Geometry check sheet. Reference: the model listing, model coordinates, mm. Face numbers are marked on the shaded views. A direction names the side the tool comes from. Coordinates: 2 decimals unless noted, no trailing zeros. Write each loop counter-clockwise with the first axis right and the second up, starting at its lowest first coordinate (ties: lowest second). Pieces come first, ordered by that corner, then holes. Notation, with made-up numbers: (-28, 35) -> (17, 35) arc R15 ccw to (17, 58) -> close; hole circle Ø10 at (-7.75, 45.25). An arc over 180 degrees is marked (long way). Answer in a Markdown table with one row per item. Add a question column.
1. Depth check by flat-ended pin: P1, Ø1.6, axis at y = 21, z = 21, coming from the +X side; P2, Ø0.6, axis at x = 15, z = 21.5, coming from the -Y side; P3, Ø0.9, axis at x = 35.5, y = 51.5, coming from the +Z side. Enter the tip coordinate at first touch or a pass-through.
2. Cross-section at A-A on z = 11. Record the cut outline in (x, y), and give its area (3 significant figures).
3. Mould release check, pull along Y, two halves, no side actions. Record for the marked faces 3, 4, 5 and 6: pulls with the +Y half, pulls with the -Y half, needs draft (parallel to the pull), parting line crosses it, or undercut.
4. Cross-section at C-C on x = 25. Record the cut outline in (y, z).
5. Set-up check for the marked faces 1 and 2: record each of +Z, -Z, +X, -X, +Y, -Y from which the full face is reachable in a straight line by a thin tool's end or side.
6. Scan lines: L1, parallel to Y at x = 15.5, z = 19.5; L2, parallel to X at y = 33, z = 15.5; L3, parallel to Y at x = 24, z = 8.5. Record each from-to range of solid material in increasing order. Write a range as from..to.
7. Cross-section at B-B on y = 23. Record the cut outline in (x, z), and give its area (3 significant figures).
8. Cross-section at D-D on y = 56. Record the cut outline in (x, z), and give its area (3 significant figures).
```python
from build123d import *

# Parameters (mm, degrees)
F0_W     = 60
F0_H     = 60
F1_DEPTH = 20
F2_W     = 48
F2_H     = 48
F3_DEPTH = 2
F5_DEPTH = 2
F6_R     = 18
F7_DEPTH = 15
F8_R     = 8.5
F9_DEPTH = 15
F10_R    = 2


with BuildPart() as f1:
    # F0 (on Top) → F1 (new body)
    with BuildSketch(Plane.XY):
        with Locations((14.998458, 30.737774)):
            Rectangle(F0_W, F0_H)
    extrude(amount=F1_DEPTH)

    # F2 (on face) → F3 (join)
    with BuildSketch(Plane.XY.offset(20)):
        with Locations((14.998458, 30.737774)):
            Rectangle(F2_W, F2_H)
    extrude(amount=F3_DEPTH)

    # F4 (on face) → F5 (cut)
    with BuildSketch(Plane.XY.offset(22)):
        with BuildLine():
            Line((-5.501542, 49.737774), (-5.501542, 51.237774))
            Line((-5.501542, 51.237774), (-4.001542, 51.237774))
            ThreePointArc((-4.001542, 51.237774), (-6.562202, 52.298434), (-5.501542, 49.737774))
        make_face()
        with BuildLine():
            Line((-4.001542, 51.237774), (-5.501542, 51.237774))
            Line((-5.501542, 51.237774), (-5.501542, 49.737774))
            ThreePointArc((-5.501542, 49.737774), (-4.440882, 50.177114), (-4.001542, 51.237774))
        make_face()
        with BuildLine():
            Line((35.498458, 51.237774), (33.998458, 51.237774))
            ThreePointArc((33.998458, 51.237774), (34.437798, 50.177114), (35.498458, 49.737774))
            Line((35.498458, 49.737774), (35.498458, 51.237774))
        make_face()
        with BuildLine():
            ThreePointArc((35.498458, 11.737774), (34.437798, 11.298434), (33.998458, 10.237774))
            Line((33.998458, 10.237774), (35.498458, 10.237774))
            Line((35.498458, 10.237774), (35.498458, 11.737774))
        make_face()
        with BuildLine():
            ThreePointArc((-4.001542, 10.237774), (-4.440882, 11.298434), (-5.501542, 11.737774))
            Line((-5.501542, 11.737774), (-5.501542, 10.237774))
            Line((-5.501542, 10.237774), (-4.001542, 10.237774))
        make_face()
        with BuildLine():
            Line((-5.501542, 10.237774), (-5.501542, 11.737774))
            ThreePointArc((-5.501542, 11.737774), (-6.562202, 9.177114), (-4.001542, 10.237774))
            Line((-4.001542, 10.237774), (-5.501542, 10.237774))
        make_face()
        with BuildLine():
            Line((35.498458, 10.237774), (33.998458, 10.237774))
            ThreePointArc((33.998458, 10.237774), (35.498458, 8.737774), (36.998458, 10.237774))
            ThreePointArc((36.998458, 10.237774), (36.559118, 11.298434), (35.498458, 11.737774))
            Line((35.498458, 11.737774), (35.498458, 10.237774))
        make_face()
        with BuildLine():
            ThreePointArc((36.998458, 51.237774), (35.498458, 52.737774), (33.998458, 51.237774))
            Line((33.998458, 51.237774), (35.498458, 51.237774))
            Line((35.498458, 51.237774), (35.498458, 49.737774))
            ThreePointArc((35.498458, 49.737774), (36.559118, 50.177114), (36.998458, 51.237774))
        make_face()
    extrude(amount=-F5_DEPTH, mode=Mode.SUBTRACT)

    # F6 (on face) → F7 (cut)
    with BuildSketch(Plane.XY.offset(22)):
        with Locations((14.998458, 30.737774)):
            Circle(F6_R)
    extrude(amount=-F7_DEPTH, mode=Mode.SUBTRACT)

    # F8 (on face) → F9 (join)
    with BuildSketch(Plane.XY.offset(7)):
        with Locations((14.998458, 30.737774)):
            Circle(F8_R)
    extrude(amount=F9_DEPTH)

    # F10
    f10_edges = [f1.edges().sort_by_distance(p)[0] for p in [
        (44.998458, 60.737774, 10),
        (44.998458, 0.737774, 10),
        (-15.001542, 0.737774, 10),
        (-15.001542, 60.737774, 10),
        (-9.001542, 54.737774, 21),
        (-9.001542, 6.737774, 21),
        (38.998458, 6.737774, 21),
        (38.998458, 54.737774, 21),
    ]]
    fillet(f10_edges, radius=F10_R)


solid = f1.part
```
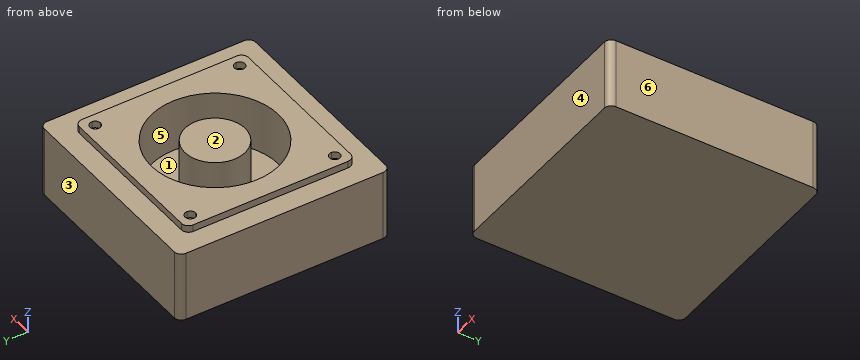
Results found:
| question | item | result |
|---|---|---|
| 1 | P1 | stops at x = 39 |
| 1 | P2 | stops at y = 6.74 |
| 1 | P3 | stops at z = 20 |
| 2 | outline | (-15, 2.74) arc R2 ccw to (-13, 0.74) -> (43, 0.74) arc R2 ccw to (45, 2.74) -> (45, 58.74) arc R2 ccw to (43, 60.74) -> (-13, 60.74) arc R2 ccw to (-15, 58.74) -> close; circle Ø17 at (15, 30.74); hole circle Ø36 at (15, 30.74) |
| 2 | area | 2,810 mm^2 |
| 3 | face 3 | pulls with the +Y half |
| 3 | face 4 | pulls with the -Y half |
| 3 | face 5 | undercut |
| 3 | face 6 | needs draft |
| 4 | outline | (0.74, 0) -> (60.74, 0) -> (60.74, 20) -> (54.74, 20) -> (54.74, 22) -> (45.7, 22) -> (45.7, 7) -> (15.77, 7) -> (15.77, 22) -> (6.74, 22) -> (6.74, 20) -> (0.74, 20) -> close |
| 5 | face 1 | +Z |
| 5 | face 2 | +Z, +X, -X, +Y, -Y |
| 6 | L1 | y = 0.74..12.74, 22.25..39.22, 48.73..60.74 |
| 6 | L2 | x = -15..-2.86, 6.81..23.19, 32.86..45 |
| 6 | L3 | y = 0.74..15.15, 46.33..60.74 |
| 7 | outline | (-15, 0) -> (45, 0) -> (45, 20) -> (39, 20) -> (39, 22) -> (31.25, 22) -> (31.25, 7) -> (18.52, 7) -> (18.52, 22) -> (11.48, 22) -> (11.48, 7) -> (-1.25, 7) -> (-1.25, 22) -> (-9, 22) -> (-9, 20) -> (-15, 20) -> close |
| 7 | area | 914 mm^2 |
| 8 | outline | (-15, 0) -> (45, 0) -> (45, 20) -> (-15, 20) -> close |
| 8 | area | 1,200 mm^2 |
